from build123d import *

# Parameters (mm, degrees)
F0_R     = 15.5
F1_DEPTH = 25
F2_T     = -3
F3_R     = 2
F4_R     = 7.5
F5_DEPTH = 15
F6_R     = 5.275719
F7_DEPTH = 10


with BuildPart() as f1:
    # F0 (on Top) → F1 (new body)
    with BuildSketch(Plane.XY):
        Circle(F0_R)
    extrude(amount=F1_DEPTH)

    # F2
    f2_openings = [f1.faces().sort_by_distance(p)[0] for p in [
        (0, 0, 0),
    ]]
    offset(amount=F2_T, openings=f2_openings)

    # F3
    f3_edges = [f1.edges().sort_by_distance(p)[0] for p in [
        (-15.5, 0, 25),
    ]]
    fillet(f3_edges, radius=F3_R)

    # F4 (on face) → F5 (join)
    with BuildSketch(Plane(origin=(0, 0, 22), x_dir=(1, 0, 0), z_dir=(0, 0, -1))):
        Circle(F4_R)
    extrude(amount=F5_DEPTH)

    # F6 (on face) → F7 (cut)
    with BuildSketch(Plane(origin=(0, 0, 7), x_dir=(1, 0, 0), z_dir=(0, 0, -1))):
        Circle(F6_R)
    extrude(amount=-F7_DEPTH, mode=Mode.SUBTRACT)


solid = f1.part
Model file for the job. Use its own axes, mm. A direction names the side the tool comes from. Give positions to 0.01 mm unless a question says otherwise; leave off trailing zeros. Order: outer loops, then holes, each group sorted by start corner. A loop starts at its lowest first (then second) coordinate and runs counter-clockwise, first axis right, second up. Notation, with made-up numbers: (65.25, 88.5) - (109.25, 88.5) arc R7 cw to (109.25, 100.5) - close; hole circle Ø3 at (43.5, 46.5). An arc over 180 degrees is marked (long way). Return JSON: item names as keys, results as strings.
1) Cut at A-A, the plane x = 0. Give the cut face in (y, z), plus the area to 3 significant figures.
Geometry says:
{"outline": "(-15.5, 0) - (-12.5, 0) - (-12.5, 22) - (-7.5, 22) - (-7.5, 7) - (-5.28, 7) - (-5.28, 17) - (5.28, 17) - (5.28, 7) - (7.5, 7) - (7.5, 22) - (12.5, 22) - (12.5, 0) - (15.5, 0) - (15.5, 23) arc R2 ccw to (13.5, 25) - (-13.5, 25) arc R2 ccw to (-15.5, 23) - close", "area": "343 mm²"}
2) Pull direction Y, two halves, no side cores. Call faces 3 (the flat face through (3, 5, 7)), 4 (the flat face through (0, 0, 25)), 5 (the cylindrical face through (-2.018, 15.368, 11.339)): pulls with the +Y half, pulls with the -Y half, needs draft (parallel to the pull), parting line crosses it, or undercut.
Geometry says:
{"face 3": "undercut", "face 4": "needs draft", "face 5": "parting line crosses it"}
3) Cut at B-B, the plane z = 8.25. Give the cut face in (x, y).
Geometry says:
{"outline": "circle Ø31 at (0, 0); circle Ø15 at (0, 0); hole circle Ø25 at (0, 0); hole circle Ø10.55 at (0, 0)"}
4) Flat gauge pins, fed straight in: P1, Ø7.5, axis at x = 1, y = 3, coming from the -Z side; P2, Ø12, axis at y = 6.5, z = 17.5, coming from the +X side; P3, Ø4, axis at x = -4, z = 7, coming from the -Y side. Where does each tip first touch, or does it go through?
Geometry says:
{"P1": "z = 7", "P2": "x = 15.49", "P3": "y = -15.37"}
5) Cut at D-D, the plane z = 19.5. Give the cut face in (x, y), plus the area to 3 significant figures.
Geometry says:
{"outline": "circle Ø31 at (0, 0); circle Ø15 at (0, 0); hole circle Ø25 at (0, 0)", "area": "441 mm²"}
6) Probe line 1 (Y direction, x = 0, z = 12); line 2 (Y direction, x = 2, z = 12); line 3 (Y direction, x = -5.5, z = 16). List the from-to ranges inside material, lowest first. Write a range as from..to.
Geometry says:
{"line 1": "-15.5..-12.5, -7.5..-5.28, 5.28..7.5, 12.5..15.5", "line 2": "-15.37..-12.34, -7.23..-4.88, 4.88..7.23, 12.34..15.37", "line 3": "-14.49..-11.22, -5.1..5.1, 11.22..14.49"}
7) 3-axis set-ups, long thin cutter, end or side, ignore diameter. For faces 1 (the flat face through (1, 13, 0)), 2 (the cylindrical face through (11.923, 3.755, 10.846)): which of +Z, -Z, +X, -X, +Y, -Y reach the whole face in a straight line?
Geometry says:
{"face 1": "-Z, +X, -X, +Y, -Y", "face 2": "-Z"}
